Verification items for the finished model (mm, model axes). Face numbers are marked on the shaded views. A direction names the side the tool comes from. Give positions to 0.01 mm unless a question says otherwise; leave off trailing zeros. Write each loop counter-clockwise with the first axis right and the second up, starting at its lowest first coordinate (ties: lowest second). Pieces come first, ordered by that corner, then holes. Notation, with made-up numbers: (-27, 25) - (19, 25) arc R26 cw to (19, 47) - close; hole circle Ø11 at (14, 78.25). An arc over 180 degrees is marked (long way). Put each result on its own line as item: value.
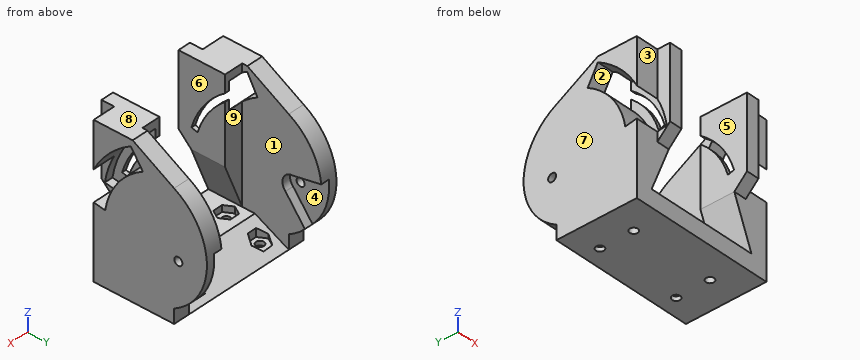
from build123d import *

# Parameters (mm, degrees)
CROQUIS1_W              = 34
CROQUIS1_H              = 19
SALIENTE_EXTRUIR1_DEPTH = 35
CROQUIS2_W              = 26.2
CROQUIS2_H              = 31
CORTAR_EXTRUIR1_DEPTH   = 25
CORTAR_EXTRUIR3_DEPTH   = 26.2
SALIENTE_EXTRUIR2_DEPTH = 34
CROQUIS10_W             = 26.2
CROQUIS10_H             = 25.966324345
CORTAR_EXTRUIR4_DEPTH   = 10
CROQUIS18_R             = 0.95
CORTAR_EXTRUIR11_DEPTH  = 4
CORTAR_EXTRUIR12_DEPTH  = 1.5
CORTAR_EXTRUIR13_DEPTH  = 3
CORTAR_EXTRUIR14_START  = -34
CROQUIS21_R             = 0.95
CORTAR_EXTRUIR14_DEPTH  = 34
SALIENTE_EXTRUIR3_DEPTH = 8
CORTAR_EXTRUIR16_START  = -34
CORTAR_EXTRUIR16_DEPTH  = 34
CROQUIS25_W             = 3
CROQUIS25_H             = 20
SALIENTE_EXTRUIR4_DEPTH = 3
CORTAR_EXTRUIR17_START  = -23.2
CORTAR_EXTRUIR17_DEPTH  = 23.2
CORTAR_EXTRUIR18_DEPTH  = 7.4
CORTAR_EXTRUIR19_START  = -7.4
CORTAR_EXTRUIR19_DEPTH  = 7.4
CORTAR_EXTRUIR20_START  = -2
CORTAR_EXTRUIR20_DEPTH  = 2
CORTAR_EXTRUIR21_DEPTH  = 28.2
CORTAR_EXTRUIR22_START  = -34
CORTAR_EXTRUIR22_DEPTH  = 34


with BuildPart() as part:
    # Croquis1 → Saliente-Extruir1 (new body)
    with BuildSketch(Plane.XY):
        with Locations((-31.887263086, 5.12254902)):
            Rectangle(CROQUIS1_W, CROQUIS1_H)
    extrude(amount=SALIENTE_EXTRUIR1_DEPTH)

    # Croquis2 → Cortar-Extruir1 (cut)
    with BuildSketch(Plane.XZ.offset(4.37745098)):
        with Locations((-31.887263086, 19.5)):
            Rectangle(CROQUIS2_W, CROQUIS2_H)
    extrude(amount=-CORTAR_EXTRUIR1_DEPTH, mode=Mode.SUBTRACT)

    # Croquis4 → Cortar-Extruir3 (cut)
    with BuildSketch(Plane.ZY.offset(18.787263086)):
        Polygon((4, 14.62254902), (4, 6.62254902), (0, 14.62254902), align=None)
    extrude(amount=CORTAR_EXTRUIR3_DEPTH, mode=Mode.SUBTRACT)

    # Croquis9 → Saliente-Extruir2 (add)
    with BuildSketch(Plane(origin=(-14.887263086, 0, 0), x_dir=(0, 0, -1), z_dir=(1, 0, 0))):
        with BuildLine():
            Line((-29.315831827, 14.62254902), (-3.349507482, 14.62254902))
            ThreePointArc((-3.349507482, 14.62254902), (-16.332669655, 22.37254902), (-29.315831827, 14.62254902))
        make_face()
    extrude(amount=-SALIENTE_EXTRUIR2_DEPTH)

    # Croquis10 → Cortar-Extruir4 (cut)
    with BuildSketch(Plane.XZ.offset(-14.62254902)):
        with Locations((-31.887263086, 16.332669655)):
            Rectangle(CROQUIS10_W, CROQUIS10_H)
    extrude(amount=-CORTAR_EXTRUIR4_DEPTH, mode=Mode.SUBTRACT)

    # Croquis18 → Cortar-Extruir11 (cut)
    with BuildSketch(Plane(origin=(0, 0, 0), x_dir=(-1, 0, 0), z_dir=(0, 0, -1))):
        with Locations((41.887263086, 2.62254902)):
            Circle(CROQUIS18_R)
        with Locations((21.887263086, 2.62254902)):
            Circle(CROQUIS18_R)
        with Locations((21.887263086, 10.62254902)):
            Circle(CROQUIS18_R)
        with Locations((41.887263086, 10.62254902)):
            Circle(CROQUIS18_R)
    extrude(amount=-CORTAR_EXTRUIR11_DEPTH, mode=Mode.SUBTRACT)

    # Croquis19 → Cortar-Extruir12 (cut)
    with BuildSketch(Plane.XY.offset(4)):
        Polygon((-43.030772734, 0.616129568), (-40.721407694, 0.629030888), (-39.577898045, 2.63545034), (-40.743753437, 4.628968471), (-43.053118477, 4.616067151), (-44.196628126, 2.609647699), align=None)
        Polygon((-23.030772734, 0.616129568), (-20.721407694, 0.629030888), (-19.577898045, 2.63545034), (-20.743753437, 4.628968471), (-23.053118477, 4.616067151), (-24.196628126, 2.609647699), align=None)
    extrude(amount=-CORTAR_EXTRUIR12_DEPTH, mode=Mode.SUBTRACT)

    # Croquis20 → Cortar-Extruir13 (cut)
    with BuildSketch(Plane.XY.offset(4)):
        Polygon((-44.081159874, 10.610292765), (-42.973597252, 8.71645054), (-40.779700463, 8.728706795), (-39.520722563, 10.735771313), (-40.628285185, 12.629613538), (-42.994825708, 12.516391244), align=None)
        Polygon((-24.081159874, 10.610292765), (-22.973597252, 8.71645054), (-20.779700463, 8.728706795), (-19.520722563, 10.735771313), (-20.628285185, 12.629613538), (-22.994825708, 12.516391244), align=None)
    extrude(amount=-CORTAR_EXTRUIR13_DEPTH, mode=Mode.SUBTRACT)

    # Croquis21 → Cortar-Extruir14 (cut)
    with BuildSketch(Plane(origin=(-14.887263086, 0, 0), x_dir=(0, 0, -1), z_dir=(1, 0, 0)).offset(CORTAR_EXTRUIR14_START)):
        with Locations((-14, 15.62254902)):
            Circle(CROQUIS21_R)
    extrude(amount=CORTAR_EXTRUIR14_DEPTH, mode=Mode.SUBTRACT)

    # Croquis23 → Saliente-Extruir3 (add)
    with BuildSketch(Plane.XZ.offset(4.37745098)):
        Polygon((-44.987263086, 35), (-40.487263086, 35), (-40.487263086, 15), (-44.987263086, 4), align=None)
        Polygon((-18.787263086, 35), (-23.287263086, 35), (-23.287263086, 15), (-18.787263086, 4), align=None)
    extrude(amount=-SALIENTE_EXTRUIR3_DEPTH)

    # Croquis24 → Cortar-Extruir16 (cut)
    with BuildSketch(Plane(origin=(-14.887263086, 0, 0), x_dir=(0, 0, -1), z_dir=(1, 0, 0)).offset(CORTAR_EXTRUIR16_START)):
        with BuildLine():
            Line((-19.364815558, -2.86477783), (-19.759303848, -4.311974772))
            ThreePointArc((-19.759303848, -4.311974772), (-26.555897405, -0.897265142), (-31.665347016, 4.737222456))
            Line((-31.665347016, 4.737222456), (-30.432986509, 5.596609942))
            ThreePointArc((-30.432986509, 5.596609942), (-25.6912281, 0.329488976), (-19.364815558, -2.86477783))
        make_face()
    extrude(amount=CORTAR_EXTRUIR16_DEPTH, mode=Mode.SUBTRACT)

    # Croquis25 → Saliente-Extruir4 (add)
    with BuildSketch(Plane.XZ.offset(4.37745098)):
        with Locations((-21.787263086, 25)):
            Rectangle(CROQUIS25_W, CROQUIS25_H)
        with Locations((-41.987263086, 25)):
            Rectangle(CROQUIS25_W, CROQUIS25_H)
    extrude(amount=SALIENTE_EXTRUIR4_DEPTH)

    # Croquis26 → Cortar-Extruir17 (cut)
    with BuildSketch(Plane(origin=(-20.287263086, 0, 0), x_dir=(0, 0, -1), z_dir=(1, 0, 0)).offset(CORTAR_EXTRUIR17_START)):
        Polygon((-18, -7.37745098), (-15, -7.37745098), (-15, -4.37745098), align=None)
    extrude(amount=CORTAR_EXTRUIR17_DEPTH, mode=Mode.SUBTRACT)

    # Croquis27 → Cortar-Extruir18 (cut)
    with BuildSketch(Plane(origin=(-14.887263086, 0, 0), x_dir=(0, 0, -1), z_dir=(1, 0, 0))):
        with BuildLine():
            Line((-16.740334426, -1.661564126), (-17.523287119, -6.599882168))
            ThreePointArc((-17.523287119, -6.599882168), (-26.750931424, -2.915621004), (-33.492032026, 4.383746258))
            Line((-33.492032026, 4.383746258), (-29.371216121, 7.25740019))
            ThreePointArc((-29.371216121, 7.25740019), (-24.094258117, 1.327236743), (-16.740334426, -1.661564126))
        make_face()
    extrude(amount=-CORTAR_EXTRUIR18_DEPTH, mode=Mode.SUBTRACT)

    # Croquis28 → Cortar-Extruir19 (cut)
    with BuildSketch(Plane.ZY.offset(48.887263086).offset(CORTAR_EXTRUIR19_START)):
        with BuildLine():
            Line((29.35443361, 7.226635221), (33.741414641, 4.827802707))
            ThreePointArc((33.741414641, 4.827802707), (26.967501757, -2.764780808), (17.541604251, -6.596970312))
            Line((17.541604251, -6.596970312), (16.754581084, -1.659299349))
            ThreePointArc((16.754581084, -1.659299349), (24.0858347, 1.321292487), (29.35443361, 7.226635221))
        make_face()
    extrude(amount=CORTAR_EXTRUIR19_DEPTH, mode=Mode.SUBTRACT)

    # Croquis29 → Cortar-Extruir20 (cut)
    with BuildSketch(Plane.ZY.offset(18.787263086).offset(CORTAR_EXTRUIR20_START)):
        with BuildLine():
            Line((17.797402962, 22.299641931), (16.5, 15.62254902))
            ThreePointArc((16.5, 15.62254902), (14.970464446, 13.318596164), (12.253440993, 13.833825555))
            Line((12.253440993, 13.833825555), (6.296886003, 18.432060872))
            ThreePointArc((6.296886003, 18.432060872), (11.631045274, 21.603150873), (17.797402962, 22.299641931))
        make_face()
    extrude(amount=CORTAR_EXTRUIR20_DEPTH, mode=Mode.SUBTRACT)

    # Croquis29<2> → Cortar-Extruir21 (cut)
    with BuildSketch(Plane.ZY.offset(18.787263086)):
        with BuildLine():
            Line((17.797402962, 22.299641931), (16.5, 15.62254902))
            ThreePointArc((16.5, 15.62254902), (14.970464446, 13.318596164), (12.253440993, 13.833825555))
            Line((12.253440993, 13.833825555), (6.296886003, 18.432060872))
            ThreePointArc((6.296886003, 18.432060872), (11.631045274, 21.603150873), (17.797402962, 22.299641931))
        make_face()
    extrude(amount=CORTAR_EXTRUIR21_DEPTH, mode=Mode.SUBTRACT)

    # Croquis30 → Cortar-Extruir22 (cut)
    with BuildSketch(Plane.ZY.offset(48.887263086).offset(CORTAR_EXTRUIR22_START)):
        Polygon((29.315831827, 14.62254902), (35, 4.827802707), (35, 14.62254902), align=None)
    extrude(amount=CORTAR_EXTRUIR22_DEPTH, mode=Mode.SUBTRACT)


solid = part.part
Q1. Section check A-A, the plane z = 7. Record the cut outline in (x, y).
Answers follow:
outline: (-48.89, -4.38) - (-43.76, -4.38) - (-43.76, 3.62) - (-44.99, 3.62) - (-44.99, 17.89) - (-46.99, 17.89) - (-46.99, 19.04) - (-48.89, 19.04) - close; (-20.01, -4.38) - (-14.89, -4.38) - (-14.89, 19.04) - (-16.79, 19.04) - (-16.79, 17.89) - (-18.79, 17.89) - (-18.79, 3.62) - (-20.01, 3.62) - close
Q2. Scan lines: line 1 along X through (y, z) = (-2.5, 25); line 2 along X through (y, z) = (-4.75, 16.5); line 3 along Z through (x, y) = (-44, -0.25). Record each from-to range of solid material in increasing order.
Answers follow:
line 1: x = -41.49 to -40.49, -23.29 to -22.29
line 2: x = -43.49 to -40.49, -23.29 to -20.29
line 3: z = 0 to 4, 6.41 to 21.37, 29.95 to 35
Q3. Section check C-C, the plane x = -29. Record the cut outline in (y, z).
Answers follow:
outline: (-4.38, 0) - (14.62, 0) - (6.62, 4) - (-4.38, 4) - close
Q4. Release check for a two-part mould opening along X. For the marked faces 6, 7, 8 and 9 record: released by +X, released by -X, zero draft, split by the parting line, or undercut.
Answers follow:
face 6: undercut
face 7: released by -X
face 8: zero draft
face 9: undercut
Q5. Go/stop test with flat-tipped pins: pin 1 Ø4.5 at (x, y) = (-41, 11) entering from +Z; pin 2 Ø4 at (x, y) = (-35.5, 9.5) entering from +Z; pin 3 Ø2.5 at (y, z) = (-6, 24.5) entering from +X. Record where each tip stops, or that it passes through.
Answers follow:
pin 1: stops at z = 2.93
pin 2: stops at z = 3.56
pin 3: stops at x = -20.29
Q6. Set-up check for the marked faces 1, 2, 3, 4 and 5: record each of +Z, -Z, +X, -X, +Y, -Y from which the full face is reachable in a straight line by a thin tool's end or side.
Answers follow:
face 1: +Z, +Y
face 2: -X
face 3: +Z, -Z, -X, -Y
face 4: +Y
face 5: +Z, +Y, -Y
Q7. Section check D-D, the plane z = 14. Record the cut outline in (x, y).
Answers follow:
outline: (-48.89, -4.38) - (-40.9, -4.38) - (-40.9, 3.62) - (-44.99, 3.62) - (-44.99, 13.12) - (-46.99, 13.12) - (-46.99, 14.67) - (-48.89, 14.67) - close; (-48.89, 16.57) - (-46.99, 16.57) - (-46.99, 22.19) - (-48.89, 22.19) - close; (-22.88, -4.38) - (-14.89, -4.38) - (-14.89, 14.67) - (-16.79, 14.67) - (-16.79, 13.12) - (-18.79, 13.12) - (-18.79, 3.62) - (-22.88, 3.62) - close; (-16.79, 16.57) - (-14.89, 16.57) - (-14.89, 22.19) - (-16.79, 22.19) - close
Q8. Section check B-B, the plane z = 22. Record the cut outline in (x, y).
Answers follow:
outline: (-48.89, 0.06) - (-41.49, 0.06) - (-41.49, -1.89) - (-40.49, -1.89) - (-40.49, 3.62) - (-44.99, 3.62) - (-44.99, 21.24) - (-48.89, 21.24) - close; (-43.49, -7.38) - (-40.49, -7.38) - (-40.49, -3.52) - (-41.49, -3.52) - (-41.49, -5.41) - (-43.49, -5.41) - close; (-23.29, -7.38) - (-20.29, -7.38) - (-20.29, -5.41) - (-22.29, -5.41) - (-22.29, -3.52) - (-23.29, -3.52) - close; (-23.29, -1.89) - (-22.29, -1.89) - (-22.29, 0.06) - (-14.89, 0.06) - (-14.89, 21.24) - (-18.79, 21.24) - (-18.79, 3.62) - (-23.29, 3.62) - close
